Autodesk Fusion 360 part; units mm, degrees
sketch "Schizzo1" plane through (0, 0, 0) normal (0, 0, 1) x (1, 0, 0)
  line L0 (0, 0) -> (35.2, 0)
  line L1 (35.2, 0) -> (35.2, 56.2)
  line L2 (35.2, 56.2) -> (0, 56.2)
  line L3 (0, 56.2) -> (0, 0)
  dimension "d1" = 35.2
  dimension "d2" = 56.2
extrude "Estrusione1" add sketch "Schizzo1" along normal blind 40
sketch "Schizzo2" plane through (0, 56.2, 0) normal (0, 1, 0) x (-1, 0, 0)
  line L0 (-35.2, 0) -> (0, 0)
  line L1 (0, 0) -> (0, 40)
  line L2 (0, 40) -> (-35.2, 40)
  line L3 (-35.2, 40) -> (-35.2, 0)
  line L4 (-35.2, 40) -> (-31.2, 40)
  line L5 (-31.2, 40) -> (-3.9522, 17.7156)
  line L6 (-3.9522, 17.7156) -> (0, 17.7156)
  dimension "d5" = 4
  dimension "d6" = 35.2
extrude "Estrusione2" cut sketch "Schizzo2" against normal blind 70 contours L1 L2 L5 L6
extrude "Estrusione3" cut 1 faces at (22.1174, 37.4667, 32.5719) along direction (0.63308, 0, -0.774086) blind 5
extrude "Estrusione4" add 1 faces at (35.2, 18.7333, 13.3333) along direction (1, 0, 0) blind 5
fillet "Raccordo1" radius 2 4 edges at (3.9522, 28.1, 17.7156) (0, 28.1, 17.7156) (31.2, 28.1, 40) (40.2, 28.1, 40)
extrude "Estrusione5" cut 1 faces at (25.2828, 37.4667, 28.7014) along direction (0.63308, 0, -0.774086) blind 3
fillet "Raccordo2" radius 1 1 edges at (36.2646, 28.1, 33.8073)
fillet "Raccordo3" radius 1 1 edges at (9.0168, 28.1, 11.5229)
sketch "Schizzo7" plane through (0, 56.2, 0) normal (0, 1, 0) x (-1, 0, 0)
  line L0 (-4.5523, 16.9817) -> (-8.3837, 12.297)
  arc A0 (-9.7909, 12.156) -> (-8.3837, 12.297) centre (-9.1578, 12.9301) ccw
  line L1 (-9.7909, 12.156) -> (-35.4906, 33.1742)
  arc A1 (-35.6316, 34.5814) -> (-35.4906, 33.1742) centre (-34.8575, 33.9483) ccw
  line L2 (-35.6316, 34.5814) -> (-33.8712, 36.7338)
  arc A2 (-33.8712, 36.7338) -> (-35.4194, 40) centre (-35.4194, 38) ccw
  line L3 (-35.4194, 40) -> (-38.2, 40)
  arc A3 (-38.2, 40) -> (-40.2, 38) centre (-38.2, 38) ccw
  line L4 (-40.2, 38) -> (-40.2, 0)
  line L5 (-40.2, 0) -> (0, 0)
  line L6 (0, 0) -> (0, 15.7156)
  arc A4 (0, 15.7156) -> (-2, 17.7156) centre (-2, 15.7156) ccw
  line L7 (-2, 17.7156) -> (-3.0042, 17.7156)
  arc A5 (-3.0042, 17.7156) -> (-4.5523, 16.9817) centre (-3.0042, 15.7156) ccw
  line L8 (-40.2, 30.6261) -> (-26, 19)
  line L9 (-26, 19) -> (-26, 7)
  line L10 (-26, 7) -> (-33, 7)
  line L11 (-33, 7) -> (-33, 2)
  line L12 (-33, 2) -> (-15, 2)
  line L13 (-15, 2) -> (-15, 7)
  line L14 (-15, 7) -> (-21, 7)
  line L15 (-21, 7) -> (-21, 16)
  line L16 (-21, 16) -> (-11, 8)
  line L17 (-11, 8) -> (-9.75, 7)
  line L18 (-9.75, 7) -> (-6, 7)
  line L19 (-6, 7) -> (0, 14.5)
extrude "Estrusione6" cut sketch "Schizzo7" against normal blind 95 contours L4 L5 L6 L8 L9 L10 L11 L12 L13 L14 L15 L16 L17 L18 L19
fillet "Raccordo4" radius 3 4 edges at (0, 28.1, 14.5) (6, 28.1, 7) (9.75, 28.1, 7) (40.2, 28.1, 30.6261)
fillet "Raccordo5" radius 1 6 edges at (26, 28.1, 7) (33, 28.1, 7) (21, 28.1, 7) (15, 28.1, 7) (15, 28.1, 2) (33, 28.1, 2)
sketch "Schizzo3" plane through (0, 56.2, 0) normal (0, 1, 0) x (-1, 0, 0)
  line L0 (-4.5523, 16.9817) -> (-8.3837, 12.297)
  arc A0 (-9.7909, 12.156) -> (-8.3837, 12.297) centre (-9.1578, 12.9301) ccw
  line L1 (-9.7909, 12.156) -> (-35.4906, 33.1742)
  arc A1 (-35.6316, 34.5814) -> (-35.4906, 33.1742) centre (-34.8575, 33.9483) ccw
  line L2 (-35.6316, 34.5814) -> (-33.8712, 36.7338)
  arc A2 (-33.8712, 36.7338) -> (-35.4194, 40) centre (-35.4194, 38) ccw
  line L3 (-35.4194, 40) -> (-38.2, 40)
  arc A3 (-38.2, 40) -> (-40.2, 38) centre (-38.2, 38) ccw
  line L4 (-40.2, 38) -> (-40.2, 0)
  line L5 (-40.2, 0) -> (0, 0)
  line L6 (0, 0) -> (0, 15.7156)
  arc A4 (0, 15.7156) -> (-2, 17.7156) centre (-2, 15.7156) ccw
  line L7 (-2, 17.7156) -> (-3.0042, 17.7156)
  arc A5 (-3.0042, 17.7156) -> (-4.5523, 16.9817) centre (-3.0042, 15.7156) ccw
  line L8 (-40.2, 29.9744) -> (-24.8148, 16.4613)
  line L9 (-24.8148, 16.4613) -> (-24.8148, 5)
  line L10 (-20.1, 5) -> (-20.1, 14)
  line L11 (-20.1, 14) -> (-8.3458, 5)
  line L12 (-8.3458, 5) -> (0, 5)
  line L13 (-32, 5) -> (-32, 0)
  line L14 (-13, 5) -> (-13, 0)
sketch "Schizzo4" plane through (0, 56.2, 0) normal (0, 1, 0) x (-1, 0, 0)
  line L0 (-24.8139, 4.9985) -> (-32, 4.9985)
sketch "Schizzo5" plane through (0, 56.2, 0) normal (0, 1, 0) x (-1, 0, 0)
  line L0 (-13, 5) -> (-20.1, 5)
sketch "Schizzo6" plane through (0, 56.2, 0) normal (0, 1, 0) x (-1, 0, 0)
  line L0 (-13, 0) -> (0, 0)
  line L1 (0, 0) -> (0, 5)
Geometry check sheet. Reference: the model listing, model coordinates, mm. A direction names the side the tool comes from. Coordinates: 2 decimals unless noted, no trailing zeros. Order: outer loops, then holes, each group sorted by start corner. A loop starts at its lowest first (then second) coordinate and runs counter-clockwise, first axis right, second up. Notation, with made-up numbers: (-18.5, -2) - (-1.5, -2) arc R12 cw to (-1.5, 10) - close; hole circle Ø2 at (8, 67.25). An arc over 180 degrees is marked (long way). Answer as a JSON object with one key per item and string values. Group by question number.
Item 1: Sectioned sample at B-B, the plane x = 18.5. Record the cut outline in (y, z).
Item 2: Sectioned sample at A-A, the plane z = 10. Record the cut outline in (x, y), and give its area (3 significant figures).
Item 3: Tool access check on faces 1 (the face through (24, 28, 2)), 2 (the face through (18, 28, 7)), 3 (the face through (3.87, 27.71, 17.52)). Record the directions out of +Z, -Z, +X, -X, +Y, -Y that give a thin tool (end or side, any length) a straight path to the whole face; none if there is none.
Item 4: Draft check along X on faces 4 (the face through (33, 28, 5)), 5 (the face through (34.74, 28.49, 35.67)), 6 (the face through (16, 28, 12)). Enter one of: +X half, -X half, draft (parallel to the pull), parting line (faces both ways), or undercut.
Item 5: Scan lines: probe 1 along X at (y, z) = (27.5, 16.5); probe 2 along Z at (x, y) = (20.5, 22); probe 3 along Z at (x, y) = (27.5, 8). Record each from-to range of solid material in increasing order.
Item 6: Sectioned sample at D-D, the plane z = 35.5. Record the cut outline in (x, y).
Item 7: Depth check by flat-ended pin: pin 1 Ø0.5 at (x, y) = (2.5, 23.5) entering from +Z; pin 2 Ø6.5 at (y, z) = (34, 10.5) entering from -X; pin 3 Ø3.5 at (y, z) = (36.5, 15.5) entering from +X. Enter the tip coordinate at first touch or a pass-through.
Resolved:
{
 "1": {"outline": "(0, 2) - (56.2, 2) - (56.2, 7) - (0, 7) - close; (0, 14) - (56.2, 14) - (56.2, 19.28) - (0, 19.28) - close"},
 "2": {"outline": "(3.6, 0) - (13.5, 0) - (13.5, 56.2) - (3.6, 56.2) - close; (21, 0) - (26, 0) - (26, 56.2) - (21, 56.2) - close", "area": "837 mm^2"},
 "3": {"face 1": "-Z, +X, -X, +Y, -Y", "face 2": "+Y, -Y", "face 3": "+Z, +Y, -Y"},
 "4": {"face 4": "+X half", "face 5": "-X half", "face 6": "undercut"},
 "5": {"probe 1": "0.16 to 4.95, 15.1 to 26", "probe 2": "2 to 7.13, 15.6 to 20.91", "probe 3": "2 to 7, 20.23 to 26.64"},
 "6": {"outline": "(34.88, 0) - (40.2, 0) - (40.2, 56.2) - (34.88, 56.2) - close"},
 "7": {"pin 1": "z = 17.72", "pin 2": "x = 0.6", "pin 3": "x = 26"}
}
